Work out the finished part from the listing and answer in its coordinate system (mm). Face numbers are marked on the shaded views. A direction names the side the tool comes from. Round coordinates to 2 decimals unless told otherwise and drop trailing zeros. Order: outer loops, then holes, each group sorted by start corner. A loop starts at its lowest first (then second) coordinate and runs counter-clockwise, first axis right, second up. Notation, with made-up numbers: (32.5, 69) - (47.5, 69) arc R28 ccw to (47.5, 98) - close; hole circle Ø1 at (-28.5, 52). An arc over 180 degrees is marked (long way). Answer in a Markdown table with one row per item.
from build123d import *

# Parameters (mm, degrees)
CUT_EXTRUDE1_DEPTH      = 54.63402325
CUT_EXTRUDE1_DEPTH_BACK = 54.63402325
SKETCH2_R               = 1.3
F7F_R                   = 0.5
FILLET2_R               = 0.5


with BuildPart() as part:
    # Sketch1 → Revolve1 (revolve)
    with BuildSketch(Plane.YZ, mode=Mode.PRIVATE) as revolve1_sk:
        Polygon((0, 0), (4.815, 0), (4.815, -2.4), (3.175, -2.4), (3.175, -53.2), (0, -53.2), align=None)
    revolve(revolve1_sk.sketch.rotate(Axis((0, 0, -335.576810525), (0, 0, 1)), 90), axis=Axis((0, 0, -335.576810525), (0, 0, 1)))

    # Sketch2 → Cut-Extrude1 (cut, two sides: drawn at the far end of the back side and taken through both)
    with BuildSketch(Plane.YZ.offset(-CUT_EXTRUDE1_DEPTH_BACK)):
        with Locations(Location((0, -47.7, 0), (0, 0, 270.000000002))):
            Circle(SKETCH2_R)
        with Locations(Location((0, -42.1, 0), (0, 0, 270.000000002))):
            Circle(SKETCH2_R)
        with Locations(Location((0, -25.3, 0), (0, 0, 270.000000002))):
            Circle(SKETCH2_R)
        with Locations(Location((0, -30.9, 0), (0, 0, 270.000000002))):
            Circle(SKETCH2_R)
        with Locations(Location((0, -36.5, 0), (0, 0, 270.000000002))):
            Circle(SKETCH2_R)
        with Locations(Location((0, -19.7, 0), (0, 0, 270.000000002))):
            Circle(SKETCH2_R)
    extrude(amount=CUT_EXTRUDE1_DEPTH + CUT_EXTRUDE1_DEPTH_BACK, mode=Mode.SUBTRACT)

    # f7f
    f7f_edges = [part.edges().sort_by_distance(p)[0] for p in [
        (4.815, 0, -2.4),
        (4.815, 0, 0),
    ]]
    fillet(f7f_edges, radius=F7F_R)

    # Fillet2
    fillet2_edges = [part.edges().sort_by_distance(p)[0] for p in [
        (3.175, 0, -53.2),
    ]]
    fillet(fillet2_edges, radius=FILLET2_R)


solid = part.part
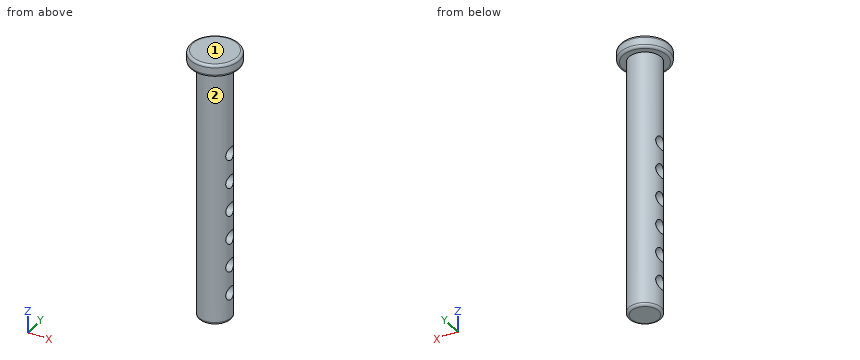
1) Find section C-C, the plane y = 0. Give the number of separate pieces and of enclosed holes in the cut face, then the cut area to 3 significant figures.
Filled in:
| item | result |
|---|---|
| separate pieces | 7 |
| enclosed holes | 0 |
| area | 246 mm^2 |
2) Find the intervals of material crossed by probe 1 along Z at (x, y) = (0.5, 3.25); probe 2 along Y at (x, z) = (1.25, -42.1); probe 3 along Y at (x, z) = (-0.75, -25.3), in increasing order. Write a range as from..to.
Filled in:
| item | result |
|---|---|
| probe 1 | z = -2.4..0 |
| probe 2 | y = -2.92..-1.3, 1.3..2.92 |
| probe 3 | y = -3.09..-1.3, 1.3..3.09 |
3) Find section B-B, the plane z = -42. Give the vertices of the cut face in (x, y) (3 decimals), then the cut area to 3 significant figures.
Filled in:
| item | result |
|---|---|
| outline | (-2.898, -1.296) arc R3.175 ccw to (2.898, -1.296) - close; (-2.898, 1.296) - (2.898, 1.296) arc R3.175 ccw to start |
| area | 15.7 mm^2 |
4) Which of the six approach directions +Z, -Z, +X, -X, +Y, -Y give full straight-line access (tool end or side, diameter ignored) to the marked faces 1 and 2?
Filled in:
| item | result |
|---|---|
| face 1 | +Z, +X, -X, +Y, -Y |
| face 2 | -Z |
5) Find section D-D, the plane z = -26. Give the vertices of the cut face in (x, y) (3 decimals).
Filled in:
| item | result |
|---|---|
| outline | (-2.98, -1.095) arc R3.175 ccw to (2.98, -1.095) - close; (-2.98, 1.095) - (2.98, 1.095) arc R3.175 ccw to start |
6) Find section A-A, the plane x = 0. Give the vertices of the cut face in (y, z) (3 decimals).
Filled in:
| item | result |
|---|---|
| outline | (-4.815, -1.9) arc R0.5 ccw to (-4.315, -2.4) - (-3.175, -2.4) - (-3.175, -52.7) arc R0.5 ccw to (-2.675, -53.2) - (2.675, -53.2) arc R0.5 ccw to (3.175, -52.7) - (3.175, -2.4) - (4.315, -2.4) arc R0.5 ccw to (4.815, -1.9) - (4.815, -0.5) arc R0.5 ccw to (4.315, 0) - (-4.315, 0) arc R0.5 ccw to (-4.815, -0.5) - close; hole circle Ø2.6 at (0, -47.7); hole circle Ø2.6 at (0, -42.1); hole circle Ø2.6 at (0, -36.5); hole circle Ø2.6 at (0, -30.9); hole circle Ø2.6 at (0, -25.3); hole circle Ø2.6 at (0, -19.7) |
7) Each of these flat-tipped pins is pushed along its axis until it touches: pin 1 (1.5 mm diameter, centred on x = 3.5, z = -31, fed in from -Y); pin 2 (1.6 mm diameter, centred on y = 0, z = -30.9, fed in from +X); pin 3 (4 mm diameter, centred on x = -0.5, z = -37, fed in from -Y) (3 decimals); pin 4 (1 mm diameter, centred on x = 2, z = -43.5, fed in from +Y). Where does it stop, or does it pass through?
Filled in:
| item | result |
|---|---|
| pin 1 | stops at y = -1.59 |
| pin 2 | passes through |
| pin 3 | stops at y = -3.175 |
| pin 4 | stops at y = 2.8 |
